Geometry: final body of the model. Coordinates: model frame, mm. A direction names the side the tool comes from. Give positions to 0.01 mm unless a question says otherwise; leave off trailing zeros. Write each loop counter-clockwise with the first axis right and the second up, starting at its lowest first coordinate (ties: lowest second). Pieces come first, ordered by that corner, then holes. Notation, with made-up numbers: M 7,35 L 50,35 A13 ccw 50,48 Z; hole C 78,37.5 d4. An arc over 180 degrees is marked long. Use one line per item in the form item = value. Start each with the question number.
Item 1: Section query A-A on z = 6. Give the number of separate pieces and of enclosed holes in the cut face, then the cut area to 3 significant figures.
Item 2: Section query C-C on x = 0. Return loops of the section in (y, z) (1 decimal).
Item 3: Access query for faces 4 (the flat face through (-17.462, 14, 6)), 5 (the flat face through (13, 24.575, 8)), 6 (the flat face through (-4.762, 4, 6)). Directions: +Z, -Z, +X, -X, +Y, -Y. A direction counts if a zero-diameter tool reaches every point of the face in a straight line with its end or side. Return the directions, or none.
Item 4: Pull-direction query (X, two-part tool) for faces 1 (the flat face through (0, 28.575, 6)), 2 (the cylindrical face through (-0.42, 22.26, 5.92)), 3 (the cylindrical face through (17.16, 28.29, 6.08)); classes: released by +X, released by -X, zero draft, split by the parting line, or undercut.
Item 5: Material intervals for line 1 along X through (y, z) = (3.75, 3.5); line 2 along Y through (x, z) = (0, 3.5) (1 decimal); line 3 along Y through (x, z) = (1, 9.25) (3 decimals), sorted ascending. Write a range as from..to.
Item 6: Section query B-B on y = 19.05. Return loops of the section in (x, z).
Item 7: Contact query for flat-ended pins moving along their axis: P1, Ø6, axis at x = 1.5, z = 8.5, coming from the -Y side; P2, Ø4, axis at x = 0, y = 19.05, coming from the +Z side; P3, Ø6, axis at x = 11.26, z = 6, coming from the +Y side (3 decimals). Output: stop coordinate, or through.
from build123d import *

# Parameters (mm, degrees)
SKETCH1_R                      = 3.2385
BOSS_EXTRUDE1_DEPTH            = 12
CBORE_FOR_M4_SHCS1_D           = 4.5
CBORE_FOR_M4_SHCS1_CBORE_D     = 8
CBORE_FOR_M4_SHCS1_CBORE_DEPTH = 4
FILLET1_R                      = 1


with BuildPart() as part:
    # Sketch1 → Boss-Extrude1 (new body)
    with BuildSketch(Plane.XY):
        Polygon((-17.4625, 28.575), (17.4625, 28.575), (17.4625, 0), (4.7625, 0), (4.7625, 9.525), (-4.7625, 9.525), (-4.7625, 0), (-17.4625, 0), align=None)
        with Locations((0, 19.05)):
            Circle(SKETCH1_R, mode=Mode.SUBTRACT)
    extrude(amount=BOSS_EXTRUDE1_DEPTH)

    # CBORE for M4 SHCS1 (through all)
    with Locations(Plane(origin=(0, 28.575, 0), x_dir=(1, 0, 0), z_dir=(0, 1, 0))):
        with Locations((-11.2625, -6), (11.2625, -6)):
            CounterBoreHole(CBORE_FOR_M4_SHCS1_D / 2, CBORE_FOR_M4_SHCS1_CBORE_D / 2, CBORE_FOR_M4_SHCS1_CBORE_DEPTH)

    # Fillet1
    fillet1_edges = [part.edges().sort_by_distance(p)[0] for p in [
        (4.7625, 9.525, 6),
        (-4.7625, 9.525, 6),
        (-17.4625, 28.575, 6),
        (17.4625, 28.575, 6),
    ]]
    fillet(fillet1_edges, radius=FILLET1_R)


solid = part.part
Answer sheet:
q1.separate_pieces = 3
q1.enclosed_holes = 1
q1.area = 589 mm2
q2.outline = M 9.5,0 L 15.8,0 L 15.8,12 L 9.5,12 Z; M 22.3,0 L 28.6,0 L 28.6,12 L 22.3,12 Z
q3.face_4 = +Z, -Z, -X, +Y, -Y
q3.face_5 = +Y
q3.face_6 = +Z, -Z, -Y
q4.face_1 = zero draft
q4.face_2 = undercut
q4.face_3 = released by +X
q5.line_1 = -17.46..-4.76, 4.76..17.46
q5.line_2 = 9.5..15.8, 22.3..28.6
q5.line_3 = 9.525..15.97, 22.13..28.575
q6.outline = M -17.46,0 L -3.24,0 L -3.24,12 L -17.46,12 Z; M 3.24,0 L 17.46,0 L 17.46,12 L 3.24,12 Z; hole C -11.26,6 d4.5; hole C 11.26,6 d4.5
q7.P1 = 9.2
q7.P2 = through
q7.P3 = 24.575
